Autodesk Inventor part; units mm, degrees
ref_plane "YZ Plane" through (0, 0, 0) normal (1, 0, 0) x (0, 1, 0)
ref_plane "XZ Plane" through (0, 0, 0) normal (0, 1, 0) x (-1, 0, 0)
ref_plane "XY Plane" through (0, 0, 0) normal (0, 0, 1) x (1, 0, 0)
sketch "Эскиз1" plane through (0, 0, 0) normal (1, 0, 0) x (0, 1, 0)
  line L0 (31, 28.4167) -> (-31, 28.4167)
  line L1 (29, -26.5833) -> (-29, -26.5833)
  line L2 (-29, -26.5833) -> (-31, 28.4167)
  line L3 (29, -26.5833) -> (31, 28.4167)
  line L4 (29, -26.5833) -> (-31, 28.4167) construction
  line L5 (31, 28.4167) -> (-29, -26.5833) construction
  line L6 (0, 39.4167) -> (0, -37.5833) construction
  point P0 (0, 0)
  point P1 (0, 0)
  point P2 (0, 0)
  point P3 (0, 28.4167)
  dimension "d0" = 58
  dimension "d1" = 62
  dimension "d2" = 55
extrude "Выдавливание1" add sketch "Эскиз1" along normal mid plane 58
sketch "Эскиз2" plane through (-29, -31, 28.4167) normal (0, 0, 1) x (1, 0, 0)
  circle A0 centre (29, 31) radius 22.5
  dimension "d5" = 45
extrude "Выдавливание2" cut sketch "Эскиз2" against normal blind 7
fillet "Сопряжение1" radius 3 2 edges at (-22.5, 0, 21.4167) (-22.5, 0, 28.4167)
sketch "Эскиз4" plane through (29, 29, -26.5833) normal (0, 0, -1) x (-1, 0, 0)
  circle A0 centre (7.95, -7.95) radius 1.5
  circle A1 centre (7.95, -50.05) radius 1.5
  circle A2 centre (50.05, -50.05) radius 1.5
  circle A3 centre (50.05, -7.95) radius 1.5
  line L0 (0, -58) -> (0, 0)
  line L1 (58, 0) -> (0, 0)
  line L2 (29, -21.9997) -> (29, -36.0003) construction
  line L3 (24.7856, -29) -> (33.2144, -29) construction
  line L4 (33.2144, -29) -> (24.7856, -29) construction
  line L5 (7.95, -7.95) -> (50.05, -7.95) construction
  line L6 (50.05, -7.95) -> (50.05, -50.05) construction
  line L7 (50.05, -50.05) -> (7.95, -50.05) construction
  line L8 (7.95, -7.95) -> (7.95, -50.05) construction
  line L9 (7.95, -7.95) -> (50.05, -50.05) construction
  line L10 (7.95, -50.05) -> (50.05, -7.95) construction
  point P0 (29, -29)
  point P1 (29, -29)
  point P2 (29, -29)
  dimension "d15" = 3
  dimension "d24" = 42.1
extrude "Выдавливание5" cut sketch "Эскиз4" against normal blind 10
properties part number "Колонка"
Part model, mm, in its own coordinate system. A direction names the side the tool comes from. Give positions to 0.01 mm unless a question says otherwise; leave off trailing zeros. Loops run counter-clockwise (first coordinate to the right, second up) from the corner with the lowest first, then second, coordinate; pieces in that order, holes last. Notation, with made-up numbers: M 57.5,5.25 L 107.5,5.25 A13 cw 107.5,17.25 Z; hole C 77,14.5 d1. An arc over 180 degrees is marked long. Put each result on its own line as item: value. Start each with the question number.
1) Probe probe 1 along X at (y, z) = (21, -24); probe 2 along Y at (x, z) = (-21.05, -21.25); probe 3 along Y at (x, z) = (-21.05, -19). List the from-to ranges inside material, lowest first.
2) Saw through at B-B (x = 0). List the corners of the cut face in (y, z), then the cut area to 4 significant figures.
3) Pull direction X, two halves, no side cores. Call faces 1 (the flat face through (0, 0, 21.417)), 2 (the flat face through (-0.406, -29.986, 0.532)), 3 (the flat face through (-29, 0, 1)), 4 (the flat face through (29, 0, 1)): +X half, -X half, draft (parallel to the pull), parting line (faces both ways), or undercut.
4) 3-axis set-ups, long thin cutter, end or side, ignore diameter. For faces 5 (the flat face through (-21, 21, -16.583)), 6 (the flat face through (-0.406, 29.986, 0.532)), 7 (the cylindrical face through (10.382, -19.961, 24.924)): which of +Z, -Z, +X, -X, +Y, -Y reach the whole face in a straight line?
5) Saw through at A-A (y = 0). List the corners of the cut face in (x, z).
6) Saw through at D-D (z = 6). List the corners of the cut face in (x, y), then the cut area to 3 significant figures.
7) Flat gauge pins, fed straight in: pin 1 (4 mm diameter, centred on x = 16.5, z = 5.5, fed in from +Y); pin 2 (1.5 mm diameter, centred on x = -20.5, y = 21.5, fed in from -Z); pin 3 (3 mm diameter, centred on x = 4, z = 15, fed in from +Y); pin 4 (3.5 mm diameter, centred on x = 20.5, y = -21, fed in from -Z). Where does each tip first touch, or does it go through?
8) Saw through at C-C (z = 23.5). List the corners of the cut face in (x, y), then the cut area to 3 significant figures.
Numbers:
1. probe 1: -29 to -22.55, -19.55 to 19.55, 22.55 to 29
1. probe 2: -29.19 to -22.55, -19.55 to 19.55, 22.55 to 29.19
1. probe 3: -29.28 to -22.55, -19.55 to 19.55, 22.55 to 29.28
2. outline: M -31,28.42 L -29,-26.58 L 29,-26.58 L 31,28.42 L 25.5,28.42 A3 ccw 22.5,25.42 L 22.5,24.42 A3 cw 19.5,21.42 L -19.5,21.42 A3 cw -22.5,24.42 L -22.5,25.42 A3 ccw -25.5,28.42 Z
2. area: 2,985 mm^2
3. face 1: undercut
3. face 2: draft
3. face 3: -X half
3. face 4: +X half
4. face 5: -Z
4. face 6: -Z, +X, -X, +Y
4. face 7: +Z
5. outline: M -29,-26.58 L 29,-26.58 L 29,28.42 L 25.5,28.42 A3 ccw 22.5,25.42 L 22.5,24.42 A3 cw 19.5,21.42 L -19.5,21.42 A3 cw -22.5,24.42 L -22.5,25.42 A3 ccw -25.5,28.42 L -29,28.42 Z
6. outline: M -29,-30.18 L 29,-30.18 L 29,30.18 L -29,30.18 Z
6. area: 3,500 mm^2
7. pin 1: y = 30.24
7. pin 2: z = -16.58
7. pin 3: y = 30.57
7. pin 4: z = -26.58
8. outline: M -29,-30.82 L 29,-30.82 L 29,30.82 L -29,30.82 Z; hole C 0,0 d44.71
8. area: 2,010 mm^2
